Can you work these out from the model? Positions are in its coordinate system, mm. A direction names the side the tool comes from. Give positions to 0.01 mm unless a question says otherwise; leave off trailing zeros. Write each loop counter-clockwise with the first axis right and the second up, starting at its lowest first coordinate (ties: lowest second). Pieces come first, ordered by that corner, then holes.
```python
from build123d import *

# Parameters (mm, degrees)
SKETCH1_W           = 38
SKETCH1_H           = 78
BOSS_EXTRUDE1_DEPTH = 16
SKETCH2_W           = 30.5
SKETCH2_H           = 70.5
CUT_EXTRUDE1_DEPTH  = 14
SKETCH3_R           = 2.75
SKETCH3_W           = 2.6
SKETCH3_H           = 5.12
SKETCH3_H_2         = 7.65
SKETCH3_H_3         = 10.2
SKETCH3_W_2         = 11
SKETCH3_H_4         = 12.5
SKETCH3_W_3         = 10.5
SKETCH3_H_5         = 14.5
SKETCH3_W_4         = 7
SKETCH3_H_6         = 5
CUT_EXTRUDE2_DEPTH  = 88.886290171
SKETCH4_W           = 11
SKETCH4_H           = 8
CUT_EXTRUDE3_DEPTH  = 3.75


with BuildPart() as part:
    # Sketch1 → Boss-Extrude1 (new body)
    with BuildSketch(Plane.XY):
        with Locations((19, 39)):
            Rectangle(SKETCH1_W, SKETCH1_H)
    extrude(amount=BOSS_EXTRUDE1_DEPTH)

    # Sketch2 → Cut-Extrude1 (cut)
    with BuildSketch(Plane.XY.offset(16)):
        with Locations((19, 39)):
            Rectangle(SKETCH2_W, SKETCH2_H)
    extrude(amount=-CUT_EXTRUDE1_DEPTH, mode=Mode.SUBTRACT)

    # Sketch3 → Cut-Extrude2 (cut, through all)
    with BuildSketch(Plane.XY.offset(2)):
        with Locations((10.05, 9.45)):
            Circle(SKETCH3_R)
        with Locations((7.25, 67.19)):
            Rectangle(SKETCH3_W, SKETCH3_H)
        with Locations((7.25, 58.805)):
            Rectangle(SKETCH3_W, SKETCH3_H_2)
        with Locations((7.25, 31.88)):
            Rectangle(SKETCH3_W, SKETCH3_H_3)
        with Locations((7.25, 18.98)):
            Rectangle(SKETCH3_W, SKETCH3_H_3)
        with Locations((22.95, 68)):
            Rectangle(SKETCH3_W_2, SKETCH3_H_4)
        with Locations((25.5, 21.5)):
            Rectangle(SKETCH3_W_3, SKETCH3_H_5)
        with Locations((22.75, 45.25)):
            Rectangle(SKETCH3_W_4, SKETCH3_H_6)
    extrude(amount=-CUT_EXTRUDE2_DEPTH, mode=Mode.SUBTRACT)

    # Sketch4 → Cut-Extrude3 (cut)
    with BuildSketch(Plane(origin=(0, 78, 0), x_dir=(1, 0, 0), z_dir=(0, 1, 0))):
        with Locations((22.95, -4)):
            Rectangle(SKETCH4_W, SKETCH4_H)
    extrude(amount=-CUT_EXTRUDE3_DEPTH, mode=Mode.SUBTRACT)


solid = part.part
```
1) Suppose I cut it at A-A on y = 9.45. Write out the boundary of the cut face in (x, z), plus the area to 3 significant figures.
Values follow:
outline: (0, 0) - (7.3, 0) - (7.3, 2) - (3.75, 2) - (3.75, 16) - (0, 16) - close; (12.8, 0) - (38, 0) - (38, 16) - (34.25, 16) - (34.25, 2) - (12.8, 2) - close
area: 170 mm2
2) For pin 1 Ø1 at (x, z) = (25.5, 0.5) entering from +Y; pin 2 Ø1 at (x, y) = (28.5, 58) entering from +Z, each with a flat end and sliding along its axis, tell me the tip position at first contact or that it passes through.
Values follow:
pin 1: stops at y = 61.75
pin 2: stops at z = 2
3) For faces 4 (the face through (23, 61.75, 1)), 5 (the face through (7, 62.63, 1)), 6 (the face through (17.45, 74, 1)), 7 (the face through (19, 39, 2)), which set-ups out of +Z, -Z, +X, -X, +Y, -Y let a thin tool reach every point of the face, with its end or its side?
Values follow:
face 4: +Z, -Z, +Y
face 5: +Z, -Z
face 6: -Z, +Y
face 7: +Z
4) If we mould it in two halves opening along X, with no side actions, what happens to faces 1 (the face through (19, 0, 8)), 2 (the face through (26.25, 45, 1)), 3 (the face through (0, 38, 8))? For each: +X half, -X half, draft (parallel to the pull), parting line (faces both ways), or undercut.
Values follow:
face 1: draft
face 2: undercut
face 3: -X half
5) Please list where these lines run through material, in increasing order: L1, parallel to X at y = 32.5, z = 13.75; L2, parallel to Y at x = 5, z = 7.5; L3, parallel to Y at x = 10.05, z = 1.65.
Values follow:
L1: x = 0 to 3.75, 34.25 to 38
L2: y = 0 to 3.75, 74.25 to 78
L3: y = 0 to 6.7, 12.2 to 78
6) Suppose I cut it at B-B on x = 30. Write out the boundary of the cut face in (y, z), plus the area to 3 significant figures.
Values follow:
outline: (0, 0) - (14.25, 0) - (14.25, 2) - (3.75, 2) - (3.75, 16) - (0, 16) - close; (28.75, 0) - (78, 0) - (78, 16) - (74.25, 16) - (74.25, 2) - (28.75, 2) - close
area: 232 mm2
7) Suppose I cut it at D-D on z = 12. Write out the boundary of the cut face in (x, y), plus the area to 3 significant figures.
Values follow:
outline: (0, 0) - (38, 0) - (38, 78) - (0, 78) - close; hole (3.75, 3.75) - (34.25, 3.75) - (34.25, 74.25) - (3.75, 74.25) - close
area: 814 mm2
8) Suppose I cut it at C-C on y = 66.5. Write out the boundary of the cut face in (x, z).
Values follow:
outline: (0, 0) - (5.95, 0) - (5.95, 2) - (3.75, 2) - (3.75, 16) - (0, 16) - close; (8.55, 0) - (17.45, 0) - (17.45, 2) - (8.55, 2) - close; (28.45, 0) - (38, 0) - (38, 16) - (34.25, 16) - (34.25, 2) - (28.45, 2) - close
